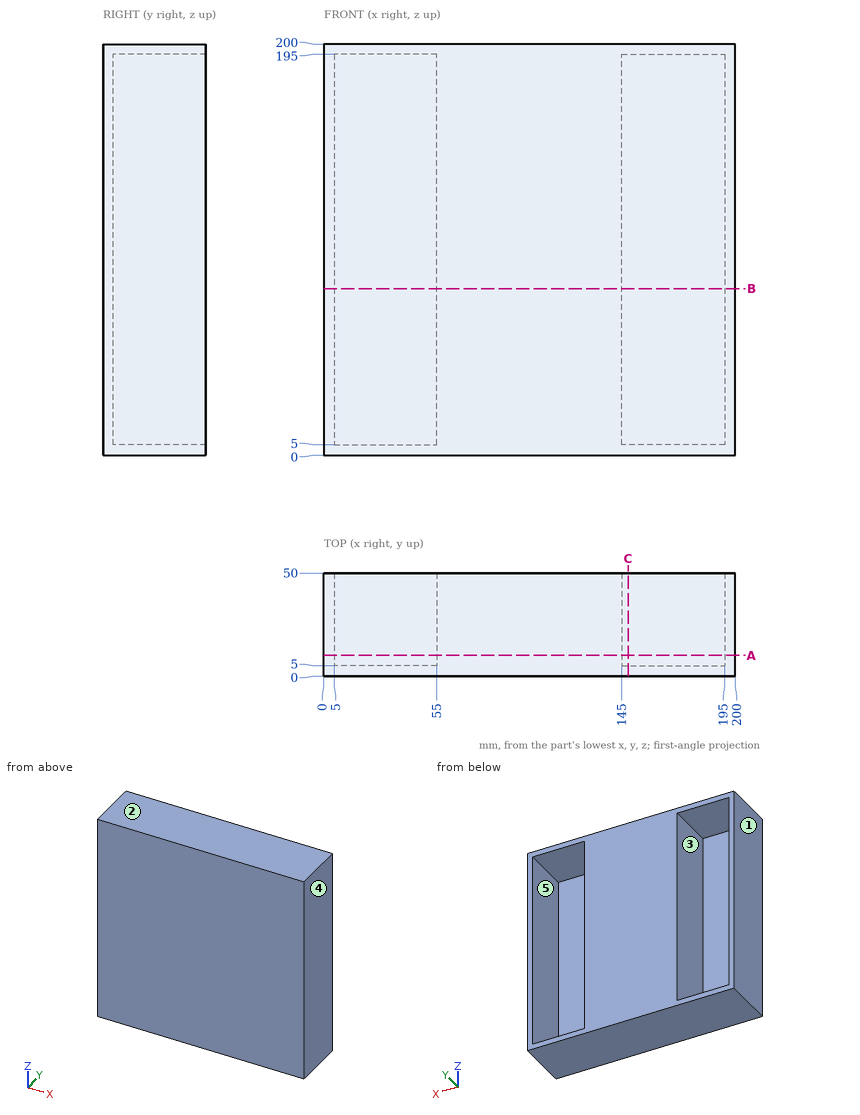
Design review of the part shown in the three views and the two pictorial views. Dimensions are in mm from the part's minimum x, y and z. A direction names the side the tool comes from. Coordinates: 2 decimals unless noted, no trailing zeros. Order: outer loops, then holes, each group sorted by start corner. A loop starts at its lowest first (then second) coordinate and runs counter-clockwise, first axis right, second up.
1) Wall thickness on line 1 along X through (y, z) = (34.5, 114.5); line 2 along Z through (x, y) = (51, 25); line 3 along Y through (x, z) = (53, 48.5): over which ranges is each line inside the solid? List them lowest first.
2) Take a section at B-B, the plane z = 81. Give the boundary of the cut face in (x, y), and give its area (3 significant figures).
3) Take a section at A-A, the plane y = 10. Give the boundary of the cut face in (x, z), and give its area (3 significant figures).
4) Take a section at C-C, the plane x = 148. Give the boundary of the cut face in (y, z), and give its area (3 significant figures).
5) For the marked faces 4 and 5, list the 3-axis set-ups (+Z, -Z, +X, -X, +Y, -Y) from which the entire face can be reached by the end or side of a thin tool; tool diameter is ignored.
6) Mouldability with a two-part tool opening along X and no side actions: class the marked faces 1, 2 and 3 as +X half, -X half, draft (parallel to the pull), parting line (faces both ways), or undercut.
Returned:
1. line 1: x = 0 to 5, 55 to 145, 195 to 200
1. line 2: z = 0 to 5, 195 to 200
1. line 3: y = 0 to 5
2. outline: (0, 0) - (200, 0) - (200, 50) - (195, 50) - (195, 5) - (145, 5) - (145, 50) - (55, 50) - (55, 5) - (5, 5) - (5, 50) - (0, 50) - close
2. area: 5,500 mm2
3. outline: (0, 0) - (200, 0) - (200, 200) - (0, 200) - close; hole (5, 5) - (55, 5) - (55, 195) - (5, 195) - close; hole (145, 5) - (195, 5) - (195, 195) - (145, 195) - close
3. area: 21,000 mm2
4. outline: (0, 0) - (50, 0) - (50, 5) - (5, 5) - (5, 195) - (50, 195) - (50, 200) - (0, 200) - close
4. area: 1,450 mm2
5. face 4: +Z, -Z, +X, +Y, -Y
5. face 5: +Y
6. face 1: -X half
6. face 2: draft
6. face 3: undercut
